```python
from build123d import *

# Parameters (mm, degrees)
ESQUISSE1_R                  = 14.12
EXTRUSION1_DEPTH             = 8
EXTRUSION2_DEPTH             = 22.511596872
R_P_TITION_CIRCULAIRE1_DEPTH = 8
ESQUISSE3_R                  = 4
EXTRUSION3_DEPTH             = 22.459027804


# Read off the part's stored shape, not the designer's step: Répétition circulaire1
with BuildPart() as part:
    # Esquisse1 → Extrusion1 (new body)
    with BuildSketch(Plane.XY):
        Circle(ESQUISSE1_R)
    extrude(amount=EXTRUSION1_DEPTH)

    # Esquisse2 → Extrusion2 (cut, through all)
    with BuildSketch(Plane.XY.offset(8)):
        Polygon((-0.5685, 13.02), (0.5685, 13.02), (2.149770097, 16.411044667), (-2.149770097, 16.411044667), align=None)
    extrude(amount=-EXTRUSION2_DEPTH, mode=Mode.SUBTRACT)

    # Répétition circulaire1 outline → Répétition circulaire1 (cut)
    with BuildSketch(Plane.XY):
        with BuildLine():
            ThreePointArc((-2.617609549, 13.875248475), (-3.654524917, 13.638872667), (-4.670707871, 13.325122438))
            Line((-4.670707871, 13.325122438), (-3.918952799, 12.429215631))
            Line((-3.918952799, 12.429215631), (-2.820695135, 12.723492885))
            Line((-2.820695135, 12.723492885), (-2.617609549, 13.875248475))
        make_face()
        with BuildLine():
            Line((3.918952799, 12.429215631), (4.670707871, 13.325122438))
            ThreePointArc((4.670707871, 13.325122438), (3.654524917, 13.638872667), (2.617609549, 13.875248475))
            Line((2.617609549, 13.875248475), (2.820695135, 12.723492885))
            Line((2.820695135, 12.723492885), (3.918952799, 12.429215631))
        make_face()
        with BuildLine():
            Line((7.002335442, 10.991400757), (7.960352825, 11.66221175))
            ThreePointArc((7.960352825, 11.66221175), (7.06, 12.228278701), (6.119595228, 12.724973644))
            Line((6.119595228, 12.724973644), (6.017664558, 11.559900757))
            Line((6.017664558, 11.559900757), (7.002335442, 10.991400757))
        make_face()
        with BuildLine():
            Line((9.608520496, 8.804540086), (10.707512889, 9.204540604))
            ThreePointArc((10.707512889, 9.204540604), (9.98434775, 9.98434775), (9.204540604, 10.707512889))
            Line((9.204540604, 10.707512889), (8.804540086, 9.608520496))
            Line((8.804540086, 9.608520496), (9.608520496, 8.804540086))
        make_face()
        with BuildLine():
            Line((11.559900757, 6.017664558), (12.724973644, 6.119595228))
            ThreePointArc((12.724973644, 6.119595228), (12.228278701, 7.06), (11.66221175, 7.960352825))
            Line((11.66221175, 7.960352825), (10.991400757, 7.002335442))
            Line((10.991400757, 7.002335442), (11.559900757, 6.017664558))
        make_face()
        with BuildLine():
            Line((12.723492885, 2.820695135), (13.875248475, 2.617609549))
            ThreePointArc((13.875248475, 2.617609549), (13.638872667, 3.654524917), (13.325122438, 4.670707871))
            Line((13.325122438, 4.670707871), (12.429215631, 3.918952799))
            Line((12.429215631, 3.918952799), (12.723492885, 2.820695135))
        make_face()
        with BuildLine():
            Line((13.02, -0.5685), (14.079948052, -1.062761894))
            ThreePointArc((14.079948052, -1.062761894), (14.12, 0), (14.079948052, 1.062761894))
            Line((14.079948052, 1.062761894), (13.02, 0.5685))
            Line((13.02, 0.5685), (13.02, -0.5685))
        make_face()
        with BuildLine():
            Line((12.429215631, -3.918952799), (13.325122438, -4.670707871))
            ThreePointArc((13.325122438, -4.670707871), (13.638872667, -3.654524917), (13.875248475, -2.617609549))
            Line((13.875248475, -2.617609549), (12.723492885, -2.820695135))
            Line((12.723492885, -2.820695135), (12.429215631, -3.918952799))
        make_face()
        with BuildLine():
            Line((10.991400757, -7.002335442), (11.66221175, -7.960352825))
            ThreePointArc((11.66221175, -7.960352825), (12.228278701, -7.06), (12.724973644, -6.119595228))
            Line((12.724973644, -6.119595228), (11.559900757, -6.017664558))
            Line((11.559900757, -6.017664558), (10.991400757, -7.002335442))
        make_face()
        with BuildLine():
            Line((8.804540086, -9.608520496), (9.204540604, -10.707512889))
            ThreePointArc((9.204540604, -10.707512889), (9.98434775, -9.98434775), (10.707512889, -9.204540604))
            Line((10.707512889, -9.204540604), (9.608520496, -8.804540086))
            Line((9.608520496, -8.804540086), (8.804540086, -9.608520496))
        make_face()
        with BuildLine():
            Line((6.017664558, -11.559900757), (6.119595228, -12.724973644))
            ThreePointArc((6.119595228, -12.724973644), (7.06, -12.228278701), (7.960352825, -11.66221175))
            Line((7.960352825, -11.66221175), (7.002335442, -10.991400757))
            Line((7.002335442, -10.991400757), (6.017664558, -11.559900757))
        make_face()
        with BuildLine():
            Line((2.820695135, -12.723492885), (2.617609549, -13.875248475))
            ThreePointArc((2.617609549, -13.875248475), (3.654524917, -13.638872667), (4.670707871, -13.325122438))
            Line((4.670707871, -13.325122438), (3.918952799, -12.429215631))
            Line((3.918952799, -12.429215631), (2.820695135, -12.723492885))
        make_face()
        with BuildLine():
            Line((-0.5685, -13.02), (-1.062761894, -14.079948052))
            ThreePointArc((-1.062761894, -14.079948052), (0, -14.12), (1.062761894, -14.079948052))
            Line((1.062761894, -14.079948052), (0.5685, -13.02))
            Line((0.5685, -13.02), (-0.5685, -13.02))
        make_face()
        with BuildLine():
            Line((-3.918952799, -12.429215631), (-4.670707871, -13.325122438))
            ThreePointArc((-4.670707871, -13.325122438), (-3.654524917, -13.638872667), (-2.617609549, -13.875248475))
            Line((-2.617609549, -13.875248475), (-2.820695135, -12.723492885))
            Line((-2.820695135, -12.723492885), (-3.918952799, -12.429215631))
        make_face()
        with BuildLine():
            Line((-7.002335442, -10.991400757), (-7.960352825, -11.66221175))
            ThreePointArc((-7.960352825, -11.66221175), (-7.06, -12.228278701), (-6.119595228, -12.724973644))
            Line((-6.119595228, -12.724973644), (-6.017664558, -11.559900757))
            Line((-6.017664558, -11.559900757), (-7.002335442, -10.991400757))
        make_face()
        with BuildLine():
            Line((-9.608520496, -8.804540086), (-10.707512889, -9.204540604))
            ThreePointArc((-10.707512889, -9.204540604), (-9.98434775, -9.98434775), (-9.204540604, -10.707512889))
            Line((-9.204540604, -10.707512889), (-8.804540086, -9.608520496))
            Line((-8.804540086, -9.608520496), (-9.608520496, -8.804540086))
        make_face()
        with BuildLine():
            Line((-11.559900757, -6.017664558), (-12.724973644, -6.119595228))
            ThreePointArc((-12.724973644, -6.119595228), (-12.228278701, -7.06), (-11.66221175, -7.960352825))
            Line((-11.66221175, -7.960352825), (-10.991400757, -7.002335442))
            Line((-10.991400757, -7.002335442), (-11.559900757, -6.017664558))
        make_face()
        with BuildLine():
            Line((-12.723492885, -2.820695135), (-13.875248475, -2.617609549))
            ThreePointArc((-13.875248475, -2.617609549), (-13.638872667, -3.654524917), (-13.325122438, -4.670707871))
            Line((-13.325122438, -4.670707871), (-12.429215631, -3.918952799))
            Line((-12.429215631, -3.918952799), (-12.723492885, -2.820695135))
        make_face()
        with BuildLine():
            Line((-13.02, 0.5685), (-14.079948052, 1.062761894))
            ThreePointArc((-14.079948052, 1.062761894), (-14.12, 0), (-14.079948052, -1.062761894))
            Line((-14.079948052, -1.062761894), (-13.02, -0.5685))
            Line((-13.02, -0.5685), (-13.02, 0.5685))
        make_face()
        with BuildLine():
            Line((-12.429215631, 3.918952799), (-13.325122438, 4.670707871))
            ThreePointArc((-13.325122438, 4.670707871), (-13.638872667, 3.654524917), (-13.875248475, 2.617609549))
            Line((-13.875248475, 2.617609549), (-12.723492885, 2.820695135))
            Line((-12.723492885, 2.820695135), (-12.429215631, 3.918952799))
        make_face()
        with BuildLine():
            Line((-10.991400757, 7.002335442), (-11.66221175, 7.960352825))
            ThreePointArc((-11.66221175, 7.960352825), (-12.228278701, 7.06), (-12.724973644, 6.119595228))
            Line((-12.724973644, 6.119595228), (-11.559900757, 6.017664558))
            Line((-11.559900757, 6.017664558), (-10.991400757, 7.002335442))
        make_face()
        with BuildLine():
            Line((-8.804540086, 9.608520496), (-9.204540604, 10.707512889))
            ThreePointArc((-9.204540604, 10.707512889), (-9.98434775, 9.98434775), (-10.707512889, 9.204540604))
            Line((-10.707512889, 9.204540604), (-9.608520496, 8.804540086))
            Line((-9.608520496, 8.804540086), (-8.804540086, 9.608520496))
        make_face()
        with BuildLine():
            Line((-6.017664558, 11.559900757), (-6.119595228, 12.724973644))
            ThreePointArc((-6.119595228, 12.724973644), (-7.06, 12.228278701), (-7.960352825, 11.66221175))
            Line((-7.960352825, 11.66221175), (-7.002335442, 10.991400757))
            Line((-7.002335442, 10.991400757), (-6.017664558, 11.559900757))
        make_face()
    extrude(amount=R_P_TITION_CIRCULAIRE1_DEPTH, mode=Mode.SUBTRACT)

    # Esquisse3 → Extrusion3 (cut, through all)
    with BuildSketch(Plane.XY.offset(8)):
        Circle(ESQUISSE3_R)
    extrude(amount=-EXTRUSION3_DEPTH, mode=Mode.SUBTRACT)


solid = part.part
```
Geometry: final body of the model. Coordinates: model frame, mm. A direction names the side the tool comes from. Coordinates: 2 decimals unless noted, no trailing zeros. Order: outer loops, then holes, each group sorted by start corner. A loop starts at its lowest first (then second) coordinate and runs counter-clockwise, first axis right, second up. Notation, with made-up numbers: M -6,80 L 7,80 A11 cw 7,94 Z; hole C -2.75,2.5 d10. An arc over 180 degrees is marked long. Answer in a Markdown table with one row per item. Add a question column.
Q1. Section query D-D on x = -5.5. Return the cut outline in (y, z).
Q2. Section query C-C on y = 10.25. Return the cut outline in (x, z).
Q3. Mould query, pull axis X, two halves, no side actions, for faces 1 (the cylindrical face through (-8.6, 11.2, 3.9)), 2 (the flat face through (-4.3, 12.883, 3.944)), 3 (the flat face through (13.02, 0, 4)). Classes: released by +X, released by -X, zero draft, split by the parting line, or undercut.
Q4. Reachability of faces 4 (the flat face through (-9.01, -10.17, 3.94)), 5 (the flat face through (9.01, 10.17, 3.94)), 6 (the flat face through (2.718, 13.307, 3.944)) from +Z, -Z, +X, -X, +Y, -Y: full face, straight path, thin tool, end or side. Return the list, or none.
Q5. Contact query for flat-ended pins moving along their axis: P1, Ø4, axis at x = -2, z = 5, coming from the +Y side; P2, Ø1.5, axis at y = -5.5, z = 1, coming from the -X side; P3, Ø0.6, axis at y = 0, z = 3.5, coming from the -X side; P4, Ø1.3, axis at x = 0, z = 3.5, coming from the -Y side. Output: stop coordinate, or through.
Q6. Line query: L1, parallel to Y at x = 0, z = 2.25; L2, parallel to X at y = -12.75, z = 4.75; L3, parallel to Y at x = -3.25, z = 1. Output: solid intervals per line, ascending.
Q7. Section query A-A on y = 0. Return the cut outline in (x, z), and give its area (3 significant figures).
Completed:
| question | item | result |
|---|---|---|
| 1 | outline | M -13,0 L 13,0 L 13,8 L -13,8 Z |
| 2 | outline | M -9.04,0 L 9.04,0 L 9.04,8 L -9.04,8 Z |
| 3 | face 1 | released by -X |
| 3 | face 2 | undercut |
| 3 | face 3 | released by +X |
| 4 | face 4 | +Z, -Z, -X |
| 4 | face 5 | +Z, -Z, +X |
| 4 | face 6 | +Z, -Z, +Y |
| 5 | P1 | stops at y = 14.08 |
| 5 | P2 | stops at x = -13.3 |
| 5 | P3 | stops at x = -13.02 |
| 5 | P4 | stops at y = -13.19 |
| 6 | L1 | y = -13.02 to -4, 4 to 13.02 |
| 6 | L2 | x = -6.07 to -4.19, -2.82 to 2.82, 4.19 to 6.07 |
| 6 | L3 | y = -12.61 to -2.33, 2.33 to 12.61 |
| 7 | outline | M -13.02,0 L -4,0 L -4,8 L -13.02,8 Z; M 4,0 L 13.02,0 L 13.02,8 L 4,8 Z |
| 7 | area | 144 mm2 |
